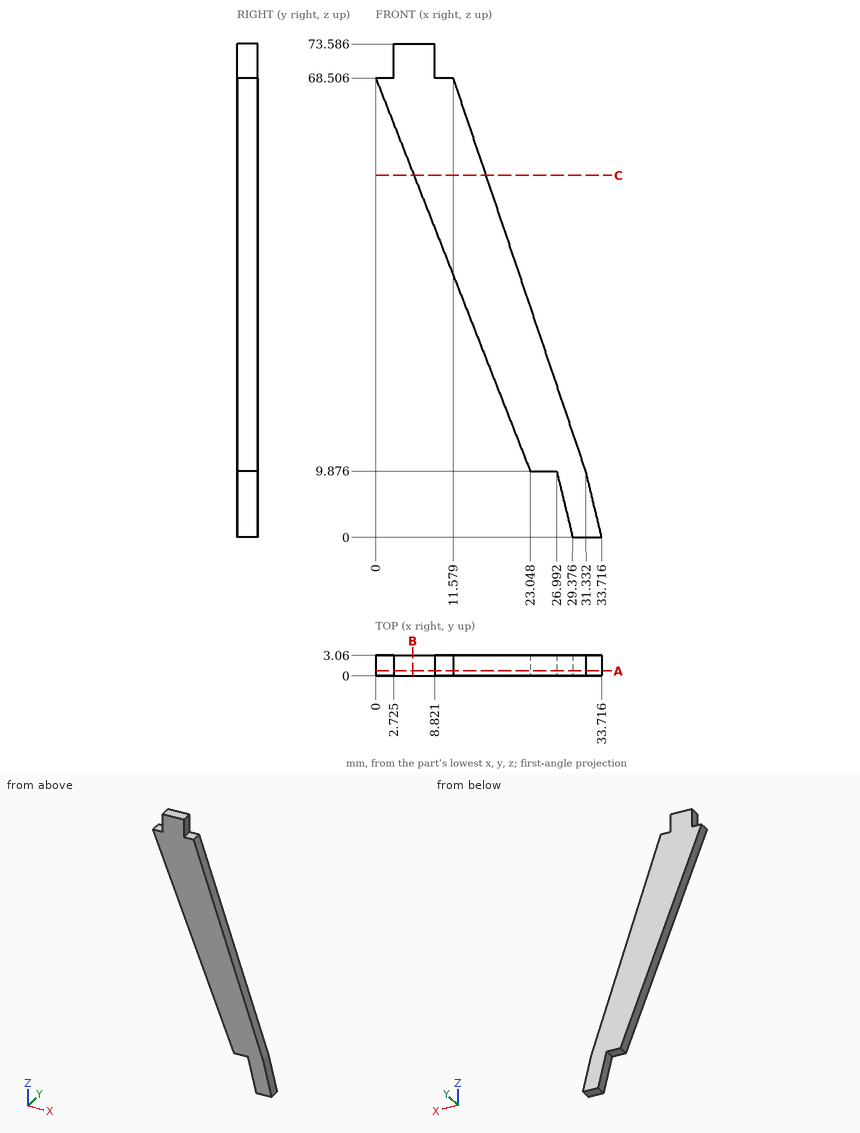
Verification items for this drawing (mm, ordinates from the low corner). Give positions to 0.01 mm unless a question says otherwise; leave off trailing zeros. Loops run counter-clockwise (first coordinate to the right, second up) from the corner with the lowest first, then second, coordinate; pieces in that order, holes last. Notation, with made-up numbers: M -6.75,6 L 29.25,6 A9 cw 29.25,13 Z; hole C 43,69.25 d8. An arc over 180 degrees is marked long. Answer as a JSON object with one key per item and string values. Group by question number.
Q1. Material ranges on line 1 along X through (y, z) = (1.2, 69) (1 decimal); line 2 along X through (y, z) = (2.4, 7.5) (1 decimal), recorded low to high. Write a range as [from, to].
Q2. Cross-section at A-A on y = 0.75. Record the cut outline in (x, z) (1 decimal).
Q3. Cross-section at C-C on z = 54. Record the cut outline in (x, y).
Q4. Go/stop test with flat-tipped pins: P1, Ø1.5, axis at y = 2.5, z = 53, coming from the -X side; P2, Ø1.4, axis at x = 10.5, y = 1.5, coming from the +Z side; P3, Ø0.9, axis at y = 1.5, z = 70.5, coming from the +X side. Record where each tip stops, or that it passes through.
Q5. Cross-section at B-B on x = 5.5. Record the cut outline in (y, z) (1 decimal).
Evaluation:
{
 "1": {"line 1": "x = [2.7, 8.8]", "line 2": "x = [27.6, 31.9]"},
 "2": {"outline": "M 0,68.5 L 23,9.9 L 27,9.9 L 29.4,0 L 33.7,0 L 31.3,9.9 L 11.6,68.5 L 8.8,68.5 L 8.8,73.6 L 2.7,73.6 L 2.7,68.5 Z"},
 "3": {"outline": "M 5.7,0 L 16.47,0 L 16.47,3.06 L 5.7,3.06 Z"},
 "4": {"P1": "stops at x = 5.8", "P2": "stops at z = 68.51", "P3": "stops at x = 8.82"},
 "5": {"outline": "M 0,54.5 L 3.1,54.5 L 3.1,73.6 L 0,73.6 Z"}
}
